```python
from build123d import *

# Parameters (mm, degrees)
MODEL_W             = 35
MODEL_H             = 35
BOSS_EXTRUDE1_DEPTH = 2
MODEL_3_R           = 1.4
CUT_EXTRUDE1_DEPTH  = 3
MODEL_4_W           = 6.9
MODEL_4_H           = 6.9
MODEL_4_R           = 0.1855
BOSS_EXTRUDE2_DEPTH = 1
BOSS_EXTRUDE3_DEPTH = 0.25


with BuildPart() as part:
    # Model → Boss-Extrude1 (new body)
    with BuildSketch(Plane.XY):
        with Locations((17.5, 17.5)):
            Rectangle(MODEL_W, MODEL_H)
    extrude(amount=-BOSS_EXTRUDE1_DEPTH)

    # Model_3 → Cut-Extrude1 (cut, through all)
    with BuildSketch(Plane.XY):
        with Locations((32.1, 32.1)):
            Circle(MODEL_3_R)
    extrude(amount=-CUT_EXTRUDE1_DEPTH, mode=Mode.SUBTRACT)

    # Model_4 → Boss-Extrude2 (add)
    with BuildSketch(Plane.XY):
        with Locations((19.35, 7.1)):
            Rectangle(MODEL_4_W, MODEL_4_H)
        with Locations((16.63, 9.82)):
            Circle(MODEL_4_R, mode=Mode.SUBTRACT)
        Polygon((3.4508, 6.65), (2.8, 6.65), (2.8, 5.9992), (2.8, 3.9008), (2.8, 3.25), (3.4508, 3.25), (5.5492, 3.25), (6.2, 3.25), (6.2, 3.9008), (6.2, 6.65), align=None)
        Polygon((5.6, 8.8508), (5.6, 8.45), (6.0008, 8.45), (9.1992, 8.45), (9.6, 8.45), (9.6, 8.8508), (9.6, 12.049229733), (9.6, 12.1), (9.25, 12.45), (9.199229733, 12.45), (6.0008, 12.45), (5.6, 12.45), (5.6, 12.0492), align=None)
    extrude(amount=BOSS_EXTRUDE2_DEPTH)

    # Model_5 → Boss-Extrude3 (add)
    with BuildSketch(Plane.XY):
        Polygon((0.25, 15.5), (0.25, 28.5), (28.75, 18.5), (31.75, 15.5), align=None)
        Polygon((0.25, 30.5), (31.75, 30.5), (31.75, 17.5), (3.25, 27.5), align=None)
    extrude(amount=BOSS_EXTRUDE3_DEPTH)


solid = part.part
```
Geometry: final body of the model. Coordinates: model frame, mm. A direction names the side the tool comes from. Coordinates: 2 decimals unless noted, no trailing zeros. Write each loop counter-clockwise with the first axis right and the second up, starting at its lowest first coordinate (ties: lowest second). Pieces come first, ordered by that corner, then holes. Notation, with made-up numbers: M 85.25,40.25 L 107.25,40.25 A16 ccw 107.25,52.25 Z; hole C 8,-12 d2. An arc over 180 degrees is marked long. Answer as CSV lines item,"result". Start each with the question number.
Q1. Cut plane B-B on x = 32.5. Return the cut outline in (y, z), then the cut area to 3 significant figures.
Q2. Cut plane C-C on y = 5.5. Return the cut outline in (x, z), then the cut area to 3 significant figures.
Q3. Reachability of faces 1 (the flat face through (4.5, 6.65, 0.5)), 2 (the flat face through (22.8, 7.1, 0.5)), 3 (the flat face through (4.5, 3.25, 0.5)) from +Z, -Z, +X, -X, +Y, -Y: full face, straight path, thin tool, end or side. Return the list, or none.
Q4. Cut plane D-D on x = 18. Return the cut outline in (y, z), then the cut area to 3 significant figures.
Q5. Line query: line 1 (X direction, y = 9.82, z = 0.45); line 2 (Y direction, x = 16.63, z = 0.8); line 3 (Z direction, x = 15, y = 14). Output: solid intervals per line, ascending. Write a range as from..to.
Q6. Pin query (flat end, axial travel): P1, Ø10.5, axis at x = 14.5, y = 18, coming from the +Z side; P2, Ø0.5, axis at y = 4, z = 0.5, coming from the -X side. Return the tip coordinate at first contact, or that it passes through.
Q7. Mould query, pull axis Y, two halves, no side actions, for faces 4 (the flat face through (17, 0, -1)), 5 (the flat face through (9.6, 10.2, 0.5)), 6 (the flat face through (7.5, 12.45, 0.5)). Classes: released by +Y, released by -Y, zero draft, split by the parting line, or undercut.
Q8. Cut plane A-A on y = 32.1. Return the cut outline in (x, z).
Findings below:
1,outline,"M 0,-2 L 30.76,-2 L 30.76,0 L 0,0 Z; M 33.44,-2 L 35,-2 L 35,0 L 33.44,0 Z"
1,area,"64.6 mm2"
2,outline,"M 0,-2 L 35,-2 L 35,0 L 22.8,0 L 22.8,1 L 15.9,1 L 15.9,0 L 6.2,0 L 6.2,1 L 2.8,1 L 2.8,0 L 0,0 Z"
2,area,"80.3 mm2"
3,face 1,"+Z, -X"
3,face 2,"+Z, +X, -Y"
3,face 3,"+Z, +X, -X, -Y"
4,outline,"M 0,-2 L 35,-2 L 35,0 L 30.5,0 L 30.5,0.25 L 22.32,0.25 L 22.32,0 L 22.27,0 L 22.27,0.25 L 15.5,0.25 L 15.5,0 L 10.55,0 L 10.55,1 L 3.65,1 L 3.65,0 L 0,0 Z"
4,area,"80.6 mm2"
5,line 1,"x = 5.6..9.6, 15.9..16.44, 16.82..22.8"
5,line 2,"y = 3.65..9.63, 10.01..10.55"
5,line 3,"z = -2..0"
6,P1,"stops at z = 0.25"
6,P2,"stops at x = 2.8"
7,face 4,"released by -Y"
7,face 5,"zero draft"
7,face 6,"undercut"
8,outline,"M 0,-2 L 30.7,-2 L 30.7,0 L 0,0 Z; M 33.5,-2 L 35,-2 L 35,0 L 33.5,0 Z"
